Build history of the part. All positions in model axes, mm. Face numbers are marked on the shaded views. A direction names the side the tool comes from. Give positions to 0.01 mm unless a question says otherwise; leave off trailing zeros. Order: outer loops, then holes, each group sorted by start corner. A loop starts at its lowest first (then second) coordinate and runs counter-clockwise, first axis right, second up. Notation, with made-up numbers: M 74,-34 L 127,-34 A19 cw 127,-29 Z; hole C 0.5,77.25 d2. An arc over 180 degrees is marked long. Use CSV: the item, a comma, the result in double quotes. Start each with the question number.
Item 1: Band-saw the part on C-C on x = -19.5. Write the cut outline in (y, z), plus the area to 3 significant figures.
Item 2: Two-plate mould, pull along X, no slides. Class the marked faces 1, 2 and 3: pulls with the +X half, pulls with the -X half, needs draft (parallel to the pull), parting line crosses it, or undercut.
Item 3: Band-saw the part on A-A on y = 6. Write the cut outline in (x, z).
Item 4: Which spindle directions (+Z, -Z, +X, -X, +Y, -Y) get a long thin tool onto all of the face, cutting with end or side? Do the marked faces 4 and 5. Say none if no direction does.
Item 5: Band-saw the part on D-D on x = -12.5. Write the cut outline in (y, z).
Item 6: Band-saw the part on B-B on z = 0. Write the cut outline in (x, y).
Item 7: Pin check, flat tips, straight feed: P1, Ø3, axis at x = -15.5, y = 8, coming from the -Z side; P2, Ø5, axis at x = -21.5, z = 3.5, coming from the -Y side. Stop position of each tip, or through.
Item 8: Wall check: line 1 along X through (y, z) = (3.75, -4.25); line 2 along X through (y, z) = (2.25, 3.75); line 3 along X through (y, z) = (8.25, 2). Give the ranges that are in metal, low to high.
from build123d import *


with BuildPart() as part:
    # Esquisse1 → Révolution2 (revolve)
    with BuildSketch(Plane.XY, mode=Mode.PRIVATE) as r_volution2_sk:
        with BuildLine():
            Line((0, 0), (-17.5, 0))
            Line((-17.5, 0), (-17.5, 2.5))
            Line((-17.5, 2.5), (-20.5, 2.5))
            Line((-20.5, 2.5), (-20.5, 0))
            Line((-20.5, 0), (-25.5, 0))
            Line((-25.5, 0), (-25.5, 1.5))
            ThreePointArc((-25.5, 1.5), (-27.5, 3.5), (-29.5, 1.5))
            Line((-29.5, 1.5), (-29.5, 0))
            Line((-29.5, 0), (-31.5, 0))
            Line((-31.5, 0), (-32, 0.5))
            Line((-32, 0.5), (-32, 6))
            Line((-32, 6), (1, 6))
            Line((1, 6), (1, 1))
            Line((1, 1), (0, 0))
        make_face()
    revolve(r_volution2_sk.sketch.rotate(Axis((-32, 6, 0), (1, 0, 0)), 270), axis=Axis((-32, 6, 0), (1, 0, 0)))


solid = part.part
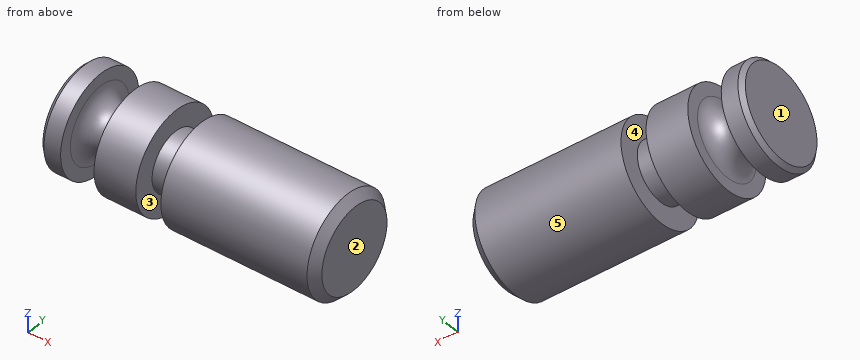
Model answer:
1,outline,"C 6,0 d7"
1,area,"38.5 mm^2"
2,face 1,"pulls with the -X half"
2,face 2,"pulls with the +X half"
2,face 3,"undercut"
3,outline,"M -32,-5.5 L -31.5,-6 L -29.5,-6 L -29.5,-4.5 A2 cw -25.5,-4.5 L -25.5,-6 L -20.5,-6 L -20.5,-3.5 L -17.5,-3.5 L -17.5,-6 L 0,-6 L 1,-5 L 1,5 L 0,6 L -17.5,6 L -17.5,3.5 L -20.5,3.5 L -20.5,6 L -25.5,6 L -25.5,4.5 A2 cw -29.5,4.5 L -29.5,6 L -31.5,6 L -32,5.5 Z"
4,face 4,"none"
4,face 5,"+X, -X"
5,outline,"C 6,0 d12"
6,outline,"M -32,0.5 L -31.5,0 L -29.5,0 L -29.5,1.5 A2 cw -25.5,1.5 L -25.5,0 L -20.5,0 L -20.5,2.5 L -17.5,2.5 L -17.5,0 L 0,0 L 1,1 L 1,11 L 0,12 L -17.5,12 L -17.5,9.5 L -20.5,9.5 L -20.5,12 L -25.5,12 L -25.5,10.5 A2 cw -29.5,10.5 L -29.5,12 L -31.5,12 L -32,11.5 Z"
7,P1,"stops at z = -5.98"
7,P2,"stops at y = 0.08"
8,line 1,"x = -32 to -29.5, -25.5 to -20.5, -17.5 to 1"
8,line 2,"x = -32 to -29.5, -25.5 to -20.5, -17.5 to 0.7"
8,line 3,"x = -32 to -28.83, -26.17 to 1"
